Input: part model. Units: mm. Frame: model coordinates. A direction names the side the tool comes from. Give positions to 0.01 mm unless a question says otherwise; leave off trailing zeros. Loops run counter-clockwise (first coordinate to the right, second up) from the corner with the lowest first, then second, coordinate; pieces in that order, holes last. Notation, with made-up numbers: (29.25, 71.5) -> (66.25, 71.5) arc R35 ccw to (66.25, 108.5) -> close; hole circle Ø8 at (74.5, 41.25). An arc over 180 degrees is marked (long way). Answer as a JSON object with one key per item and string values.
```python
from build123d import *

# Parameters (mm, degrees)
F0_R     = 11
F0_R_2   = 9.5
F1_DEPTH = 3
F0_W     = 44
F0_H     = 3
F2_DEPTH = 15
F3_DEPTH = 25
F5_DEPTH = 50


with BuildPart() as f1:
    # F0 (on Top) → F1 (new body)
    with BuildSketch(Plane.XY):
        with BuildLine():
            Line((22, -30), (22, 0))
            ThreePointArc((22, 0), (0, -22), (-22, 0))
            Line((-22, 0), (-22, -30))
            Line((-22, -30), (22, -30))
        make_face()
        with BuildLine():
            ThreePointArc((-22, 0), (0, -22), (22, 0))
            ThreePointArc((22, 0), (0, 22), (-22, 0))
        make_face()
        Circle(F0_R, mode=Mode.SUBTRACT)
        Circle(F0_R)
        Circle(F0_R_2, mode=Mode.SUBTRACT)
    extrude(amount=F1_DEPTH)

    # F0 (on Top) → F2 (join)
    with BuildSketch(Plane.XY):
        with Locations((0, -31.5)):
            Rectangle(F0_W, F0_H)
    extrude(amount=F2_DEPTH)

    # F0 (on Top) → F3 (join)
    with BuildSketch(Plane.XY):
        Circle(F0_R)
        Circle(F0_R_2, mode=Mode.SUBTRACT)
    extrude(amount=-F3_DEPTH)

    # F4 (on Front) → F5 (cut)
    with BuildSketch(Plane.XZ):
        with BuildLine():
            ThreePointArc((-18.249251, 10.8364), (-16.097239, 8.645825), (-13.919441, 10.810768))
            ThreePointArc((-13.919441, 10.810768), (-13.91963, 10.839348), (-13.920196, 10.867923))
            ThreePointArc((-13.920196, 10.867923), (-16.100186, 12.975691), (-18.249251, 10.8364))
        make_face()
        with BuildLine():
            ThreePointArc((-13.920196, 10.867923), (-13.91963, 10.839348), (-13.919441, 10.810768))
            ThreePointArc((-13.919441, 10.810768), (-16.097239, 8.645825), (-18.249251, 10.8364))
            Line((-18.249251, 10.8364), (-18.308776, 5.809141))
            ThreePointArc((-18.308776, 5.809141), (-16.064272, 8.043438), (-13.787468, 5.842063))
            Line((-13.787468, 5.842063), (-13.920196, 10.867923))
        make_face()
        with BuildLine():
            ThreePointArc((-13.78668, 5.78237), (-13.786877, 5.812219), (-13.787468, 5.842063))
            ThreePointArc((-13.787468, 5.842063), (-16.064272, 8.043438), (-18.308776, 5.809141))
            ThreePointArc((-18.308776, 5.809141), (-16.061193, 3.521282), (-13.78668, 5.78237))
        make_face()
        with BuildLine():
            ThreePointArc((18.249403, 10.810768), (16.055842, 8.645976), (13.920196, 10.867923))
            Line((13.920196, 10.867923), (13.787468, 5.842063))
            ThreePointArc((13.787468, 5.842063), (16.064272, 8.043438), (18.308776, 5.809141))
            Line((18.308776, 5.809141), (18.249251, 10.8364))
            ThreePointArc((18.249251, 10.8364), (18.249365, 10.823584), (18.249403, 10.810768))
        make_face()
        with BuildLine():
            ThreePointArc((18.249251, 10.8364), (16.100186, 12.975691), (13.920196, 10.867923))
            ThreePointArc((13.920196, 10.867923), (16.055842, 8.645976), (18.249403, 10.810768))
            ThreePointArc((18.249403, 10.810768), (18.249365, 10.823584), (18.249251, 10.8364))
        make_face()
        with BuildLine():
            ThreePointArc((18.308776, 5.809141), (16.064272, 8.043438), (13.787468, 5.842063))
            ThreePointArc((13.787468, 5.842063), (16.017958, 3.52144), (18.308935, 5.78237))
            ThreePointArc((18.308935, 5.78237), (18.308895, 5.795756), (18.308776, 5.809141))
        make_face()
    extrude(amount=F5_DEPTH, mode=Mode.SUBTRACT)


solid = f1.part
```
Q1. Section B-B, the plane y = -7. Return the cut outline in (x, z).
Evaluation:
{"outline": "(-22, 0) -> (-8.49, 0) -> (-8.49, -25) -> (-6.42, -25) -> (-6.42, 3) -> (-22, 3) -> close; (6.42, -25) -> (8.49, -25) -> (8.49, 0) -> (22, 0) -> (22, 3) -> (6.42, 3) -> close"}
Q2. Draft query along Z for faces 1 (the flat face through (22, -20, 2)), 2 (the flat face through (0, -31, 15)), 3 (the cylindrical face through (-16.111, -31.479, 3.522)). Return one class per face: +Z half, -Z half, draft (parallel to the pull), parting line (faces both ways), or undercut.
Evaluation:
{"face 1": "draft", "face 2": "+Z half", "face 3": "undercut"}
Q3. Section C-C, the plane z = -22. Return the cut outline in (x, y), then the cut area to 3 significant figures.
Evaluation:
{"outline": "circle Ø22 at (0, 0); hole circle Ø19 at (0, 0)", "area": "96.6 mm2"}
Q4. Pin query (flat end, axial travel): pin 1 (22 mm diameter, centred on x = -5, y = -12, fed in from +Z); pin 2 (1.5 mm diameter, centred on x = 17, y = -11.5, fed in from -Z); pin 3 (5 mm diameter, centred on x = -6, z = -17.5, fed in from +Y); pin 4 (8 mm diameter, centred on x = -4, y = 1, fed in from -Z). Return the tip coordinate at first contact, or that it passes through.
Evaluation:
{"pin 1": "stops at z = 3", "pin 2": "stops at z = 0", "pin 3": "stops at y = 10.43", "pin 4": "passes through"}
Q5. Access query for faces 4 (the flat face through (-22, -20, 2)), 5 (the cylindrical face through (16.147, -31.479, 12.975)), 6 (the flat face through (-5, -9, 3)), 7 (the cylindrical face through (-2.38, -10.74, -12.32)). Directions: +Z, -Z, +X, -X, +Y, -Y. A direction counts if a zero-diameter tool reaches every point of the face in a straight line with its end or side. Return the directions, or none.
Evaluation:
{"face 4": "+Z, -Z, -X, +Y, -Y", "face 5": "+Y, -Y", "face 6": "+Z, +X, -X, +Y", "face 7": "-Z"}
Q6. Ray query, line 1 along Y through (x, z) = (0, 1.9); line 2 along Y through (x, z) = (0, -10); line 3 along Z through (x, y) = (-4.5, -18.5). Return the intervals inside material, ascending.
Evaluation:
{"line 1": "y = -33 to -9.5, 9.5 to 22", "line 2": "y = -11 to -9.5, 9.5 to 11", "line 3": "z = 0 to 3"}
Q7. Section A-A, the plane x = 0. Return the cut outline in (y, z).
Evaluation:
{"outline": "(-33, 0) -> (-11, 0) -> (-11, -25) -> (-9.5, -25) -> (-9.5, 3) -> (-30, 3) -> (-30, 15) -> (-33, 15) -> close; (9.5, -25) -> (11, -25) -> (11, 0) -> (22, 0) -> (22, 3) -> (9.5, 3) -> close"}
Q8. Section D-D, the plane y = -23.5. Return the cut outline in (x, z).
Evaluation:
{"outline": "(-22, 0) -> (22, 0) -> (22, 3) -> (-22, 3) -> close"}
